from build123d import *

# Parameters (mm, degrees)
F0_W      = 140
F0_H      = 110
F0_W_2    = 35
F0_H_2    = 25
F1_DEPTH  = 4.826
F2_W      = 31.75
F2_H      = 31.75
F2_W_2    = 25.4
F2_H_2    = 25.4
F3_DEPTH  = 120
F4_W      = 6
F4_H      = 31.75
F4_W_2    = 2.825
F4_H_2    = 25.4
F5_DEPTH  = 110
F6_R      = 3
F7_DEPTH  = 10
F8_W      = 25.4
F8_H      = 25.4
F8_W_2    = 15.874
F8_H_2    = 15.874
F9_DEPTH  = 20
F11_DEPTH = 152


with BuildPart() as f1:
    # F0 (on Top) → F1 (new body)
    with BuildSketch(Plane.XY):
        with Locations((3.5, 55)):
            Rectangle(F0_W, F0_H)
        with BuildLine():
            Line((-66.5, 210), (-66.5, 110))
            Line((-66.5, 110), (73.5, 110))
            Line((73.5, 110), (73.5, 210))
            Line((73.5, 210), (38.5, 210))
            add(Edge.make_bspline(
                [(-31.5, 210), (-31.5, 178), (-26.1927577262, 110.7427430843), (33.1927577262, 110.7427430843), (38.5, 178), (38.5, 210)],
                knots=[0, 0, 0, 0, 0.3861272069, 0.6138727931, 1, 1, 1, 1], degree=3))
            Line((-31.5, 210), (-66.5, 210))
        make_face()
        with Locations((-49, 222.5)):
            Rectangle(F0_W_2, F0_H_2)
        with Locations((56, 222.5)):
            Rectangle(F0_W_2, F0_H_2)
    extrude(amount=F1_DEPTH)

    # F2 (on face) → F3 (join)
    with BuildSketch(Plane.XZ):
        with Locations((-50.625, -15.875)):
            Rectangle(F2_W, F2_H)
        with Locations((-50.625, -15.875)):
            Rectangle(F2_W_2, F2_H_2, mode=Mode.SUBTRACT)
        with Locations((57.625, -15.875)):
            Rectangle(F2_W, F2_H)
        with Locations((57.625, -15.875)):
            Rectangle(F2_W_2, F2_H_2, mode=Mode.SUBTRACT)
    extrude(amount=-F3_DEPTH)

    # F4 (on face) → F5 (join)
    with BuildSketch(Plane(origin=(0, 120, 0), x_dir=(-1, 0, 0), z_dir=(0, 1, 0))):
        with Locations((63.5, -15.875)):
            Rectangle(F4_W, F4_H)
        with Locations((-68.9125, -15.875)):
            Rectangle(F4_W_2, F4_H_2)
        Polygon((-67.5, 0), (-73.5, 0), (-73.5, -31.75), (-70.325, -31.75), (-67.5, -31.75), (-67.5, -28.575), (-70.325, -28.575), (-70.325, -3.175), (-67.5, -3.175), align=None)
    extrude(amount=F5_DEPTH)

    # F6 (on face) → F7 (cut)
    with BuildSketch(Plane.YZ.offset(-34.75)):
        with Locations((60, -10)):
            Circle(F6_R)
    extrude(amount=-F7_DEPTH, mode=Mode.SUBTRACT)

    # F8 (on face) → F9 (join, symmetric)
    with BuildSketch(Plane.XZ):
        with Locations((-50.625, -15.875)):
            Rectangle(F8_W, F8_H)
        with Locations((-50.625, -15.875)):
            Rectangle(F8_W_2, F8_H_2, mode=Mode.SUBTRACT)
        with Locations((57.625, -15.875)):
            Rectangle(F8_W, F8_H)
        with Locations((57.625, -15.875)):
            Rectangle(F8_W_2, F8_H_2, mode=Mode.SUBTRACT)
    extrude(amount=F9_DEPTH, both=True)

    # F10 (on face) → F11 (cut)
    with BuildSketch(Plane(origin=(-66.5, 0, 0), x_dir=(0, -1, 0), z_dir=(-1, 0, 0))):
        with BuildLine():
            ThreePointArc((-180, -21), (-176.8180194847, -19.6819805153), (-175.5, -16.5))
            ThreePointArc((-175.5, -16.5), (-176.8180194847, -13.3180194847), (-180, -12))
            Line((-180, -12), (-180, -16.5))
            Line((-180, -16.5), (-180, -21))
        make_face()
        with BuildLine():
            Line((-180, -16.5), (-180, -12))
            ThreePointArc((-180, -12), (-184.5, -16.5), (-180, -21))
            Line((-180, -21), (-180, -16.5))
        make_face()
        with BuildLine():
            ThreePointArc((-180, -21), (-184.5, -16.5), (-180, -12))
            Line((-180, -12), (-230, -12))
            Line((-230, -12), (-230, -21))
            Line((-230, -21), (-180, -21))
        make_face()
    extrude(amount=-F11_DEPTH, mode=Mode.SUBTRACT)


solid = f1.part
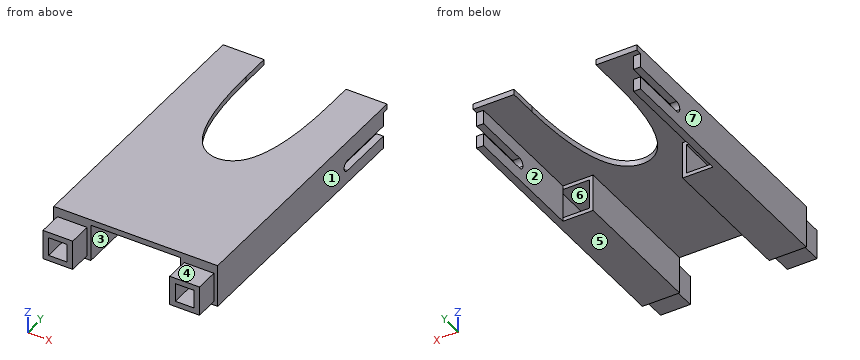
The model under review builds one solid part; all positions refer to its coordinate system, in mm. Face numbers are marked on the shaded views. A direction names the side the tool comes from. Round coordinates to 2 decimals unless told otherwise and drop trailing zeros. Write each loop counter-clockwise with the first axis right and the second up, starting at its lowest first coordinate (ties: lowest second). Pieces come first, ordered by that corner, then holes. Notation, with made-up numbers: (64.25, 68.5) - (84.25, 68.5) arc R30 ccw to (84.25, 96.5) - close; hole circle Ø5 at (58.5, -31). An arc over 180 degrees is marked (long way). One line per item, written item: value. Start each with the question number.
1. Clearance check with flat-ended pins moving along their axes: P1, Ø7.5, axis at x = 57, z = -15.5, coming from the +Y side; P2, Ø22, axis at x = -49, y = -12.5, coming from the +Z side (3 decimals); P3, Ø5, axis at x = 39, z = -2, coming from the -Y side; P4, Ø4, axis at x = -30.5, y = 101.5, coming from the -Z side. State where each tip first meets the part, or that it passes through.
2. Consider section B-B on y = 60. Write out the cut boundary in (x, z) (3 decimals).
3. Consider section C-C on y = 17.5. Write out the cut boundary in (x, z).
4. The part is to be moulded in two halves that separate along Z. For the marked faces 5, 6 and 7, say which applies: released by +Z, released by -Z, zero draft, split by the parting line, or undercut.
5. To check wall thickness, follow L1, parallel to X at y = 96.5, z = -15.5 (3 decimals); L2, parallel to X at y = 10, z = -21.5; L3, parallel to X at y = 142.5, z = -11. State the ranges of each line that lie inside material, in increasing order. Write a range as from..to.
6. Consider section A-A on y = 109. Write out the cut boundary in (x, z) (3 decimals).
7. Machinability: for the marked faces 1, 2, 3 and 4, which of the approach directions +Z, -Z, +X, -X, +Y, -Y give a long, thin tool a straight path to every point of the face, cutting with its end or side? Answer none if there is none.
Checks:
1. P1: passes through
1. P2: stops at z = -3.175
1. P3: stops at y = 0
1. P4: stops at z = 0
2. outline: (-66.5, -31.75) - (-34.75, -31.75) - (-34.75, -13) - (-37.925, -13) - (-37.925, -28.575) - (-63.325, -28.575) - (-63.325, -3.175) - (-37.925, -3.175) - (-37.925, -7) - (-34.75, -7) - (-34.75, 0) - (41.75, 0) - (41.75, -31.75) - (73.5, -31.75) - (73.5, 4.826) - (-66.5, 4.826) - close; hole (44.925, -28.575) - (70.325, -28.575) - (70.325, -3.175) - (44.925, -3.175) - close
3. outline: (-66.5, -31.75) - (-34.75, -31.75) - (-34.75, 0) - (41.75, 0) - (41.75, -31.75) - (73.5, -31.75) - (73.5, 4.83) - (-66.5, 4.83) - close; hole (-58.56, -23.81) - (-42.69, -23.81) - (-42.69, -7.94) - (-58.56, -7.94) - close; hole (49.69, -23.81) - (65.56, -23.81) - (65.56, -7.94) - (49.69, -7.94) - close
4. face 5: released by -Z
4. face 6: undercut
4. face 7: zero draft
5. L1: x = -66.5..-63.325, -37.925..-34.75, 41.75..44.925, 70.325..73.5
5. L2: x = -66.5..-58.56, -42.69..-34.75, 41.75..49.69, 65.56..73.5
5. L3: x = -66.5..-60.5, 67.5..73.5
6. outline: (-66.5, -31.75) - (-34.75, -31.75) - (-34.75, 0) - (41.75, 0) - (41.75, -31.75) - (73.5, -31.75) - (73.5, 4.826) - (-66.5, 4.826) - close; hole (-63.325, -28.575) - (-37.925, -28.575) - (-37.925, -3.175) - (-63.325, -3.175) - close; hole (44.925, -28.575) - (70.325, -28.575) - (70.325, -3.175) - (44.925, -3.175) - close
7. face 1: +Z, -Z, +X, +Y, -Y
7. face 2: -Z, +Y
7. face 3: -Z, +Y, -Y
7. face 4: +Z, +X, -X, -Y
